```python
from build123d import *

# Parameters (mm, degrees)
F1_DEPTH = 152.4
F2_R     = 38.1
F3_DEPTH = 152.4
F5_DEPTH = 127
F7_DEPTH = 25.4


with BuildPart() as f1:
    # F0 (on Front) → F1 (new body)
    with BuildSketch(Plane.XZ):
        with BuildLine():
            Line((0, 50.8), (0, 0))
            Line((0, 0), (127, 0))
            Line((127, 0), (127, 154.6394254648))
            ThreePointArc((127, 154.6394254648), (84.2300226684, 178.0283138665), (80.8435975712, 226.6579672344))
            Line((80.8435975712, 226.6579672344), (0, 50.8))
        make_face()
        with BuildLine():
            Line((127, 154.6394254648), (127, 0))
            Line((127, 0), (254, 0))
            Line((254, 0), (254, 50.8))
            Line((254, 50.8), (173.1564024288, 226.6579672344))
            ThreePointArc((173.1564024288, 226.6579672344), (176.6255238934, 216.2997835762), (177.8, 205.4394254648))
            ThreePointArc((177.8, 205.4394254648), (162.9210244843, 169.5184009805), (127, 154.6394254648))
        make_face()
        with BuildLine():
            ThreePointArc((80.8435975712, 226.6579672344), (84.2300226684, 178.0283138665), (127, 154.6394254648))
            ThreePointArc((127, 154.6394254648), (162.9210244843, 169.5184009805), (177.8, 205.4394254648))
            ThreePointArc((177.8, 205.4394254648), (176.6255238934, 216.2997835762), (173.1564024288, 226.6579672344))
            ThreePointArc((173.1564024288, 226.6579672344), (127, 256.2394254648), (80.8435975712, 226.6579672344))
        make_face()
    extrude(amount=F1_DEPTH)

    # F2 (on face) → F3 (cut)
    with BuildSketch(Plane(origin=(0, 0, 0), x_dir=(-1, 0, 0), z_dir=(0, 1, 0))):
        with Locations((-127, 205.4394254648)):
            Circle(F2_R)
    extrude(amount=-F3_DEPTH, mode=Mode.SUBTRACT)

    # F4 (on face) → F5 (cut)
    with BuildSketch(Plane(origin=(0, 0, 0), x_dir=(-1, 0, 0), z_dir=(0, 1, 0))):
        with BuildLine():
            Line((-173.1564024288, 226.6579672344), (-254, 50.8))
            Line((-254, 50.8), (-139.7, 50.8))
            Line((-139.7, 50.8), (-139.7, 156.2525369679))
            ThreePointArc((-139.7, 156.2525369679), (-172.8830053448, 183.6359894848), (-173.1564024288, 226.6579672344))
        make_face()
        with BuildLine():
            Line((0, 50.8), (-80.8435975712, 226.6579672344))
            ThreePointArc((-80.8435975712, 226.6579672344), (-77.3744761066, 216.2997835762), (-76.2, 205.4394254648))
            ThreePointArc((-76.2, 205.4394254648), (-86.8390737159, 174.3309057314), (-114.3, 156.2525369679))
            Line((-114.3, 156.2525369679), (-114.3, 109.0697127324))
            Line((-114.3, 109.0697127324), (-114.3, 50.8))
            Line((-114.3, 50.8), (0, 50.8))
        make_face()
    extrude(amount=-F5_DEPTH, mode=Mode.SUBTRACT)

    # F6 (on face) → F7 (cut)
    with BuildSketch(Plane(origin=(0, 0, 0), x_dir=(-1, 0, 0), z_dir=(0, 1, 0))):
        with BuildLine():
            ThreePointArc((-114.3, 156.2525369679), (-127, 154.6394254648), (-139.7, 156.2525369679))
            Line((-139.7, 156.2525369679), (-139.7, 50.8))
            Line((-139.7, 50.8), (-114.3, 50.8))
            Line((-114.3, 50.8), (-114.3, 156.2525369679))
        make_face()
    extrude(amount=-F7_DEPTH, mode=Mode.SUBTRACT)


solid = f1.part
```
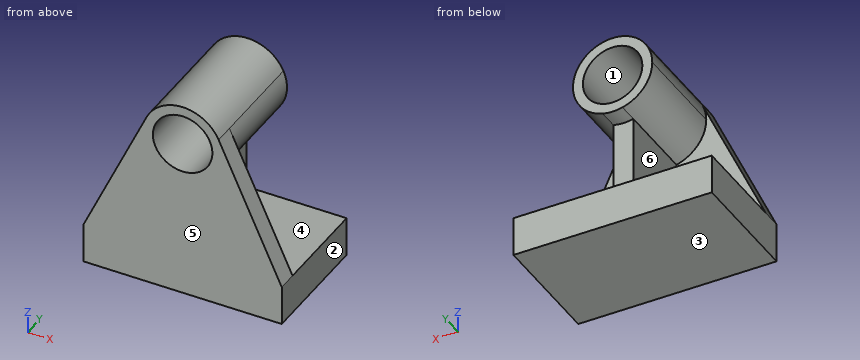
CAD build for the part. Positions are in the model's coordinates, mm. Face numbers are marked on the shaded views. A direction names the side the tool comes from. Coordinates: 2 decimals unless noted, no trailing zeros. Order: outer loops, then holes, each group sorted by start corner. A loop starts at its lowest first (then second) coordinate and runs counter-clockwise, first axis right, second up. Notation, with made-up numbers: (14.25, 16.25) -> (60.25, 16.25) arc R22 ccw to (60.25, 41.25) -> close; hole circle Ø2 at (41.25, 56.25). An arc over 180 degrees is marked (long way). Use one line per item in the form item = value. Start each with the question number.
1) Band-saw the part on A-A on x = 127. Give the cut face in (y, z), then the cut area to 3 significant figures.
2) Pull direction Z, two halves, no side cores. Call the marked faces 1, 2 and 3: +Z half, -Z half, draft (parallel to the pull), parting line (faces both ways), or undercut.
3) Band-saw the part on C-C on z = 197.5. Give the cut face in (x, y), then the cut area to 3 significant figures.
4) Band-saw the part on B-B on y = -136. Give the cut face in (x, z), then the cut area to 3 significant figures.
5) Drop flat-ended pins along their axis: pin 1 (3 mm diameter, centred on y = -73, z = 196, fed in from +X); pin 2 (4 mm diameter, centred on x = 132.5, z = 88, fed in from +Y); pin 3 (4 mm diameter, centred on x = 184, y = -60.5, fed in from +Z). Give the stop position or say it passes through.
6) Band-saw the part on D-D on y = -79. Give the cut face in (x, z), then the cut area to 3 significant figures.
7) Tool access for the marked faces 4, 5 and 6: list every direction of +Z, -Z, +X, -X, +Y, -Y with a clear straight run to the whole face (end or side of a thin tool).
8) Drill centre lines: L1, parallel to Z at x = 127, y = -45; L2, parallel to Z at x = 100.5, y = -103.5; L3, parallel to Z at x = 109.5, y = -124.5. Where is each one in solid material? Low to high. Write a range as [from, to].
Entries:
q1.outline = (-152.4, 0) -> (0, 0) -> (0, 50.8) -> (-25.4, 50.8) -> (-25.4, 154.64) -> (0, 154.64) -> (0, 167.34) -> (-152.4, 167.34) -> close; (-152.4, 243.54) -> (0, 243.54) -> (0, 256.24) -> (-152.4, 256.24) -> close
q1.area = 24,800 mm2
q2.face_1 = undercut
q2.face_2 = draft
q2.face_3 = -Z half
q3.outline = (67.44, -152.4) -> (89.74, -152.4) -> (89.74, 0) -> (76.82, 0) -> (76.82, -127) -> (67.44, -127) -> close; (164.26, -152.4) -> (186.56, -152.4) -> (186.56, -127) -> (177.18, -127) -> (177.18, 0) -> (164.26, 0) -> close
q3.area = 4,410 mm2
q4.outline = (0, 0) -> (254, 0) -> (254, 50.8) -> (173.16, 226.66) arc R50.8 ccw to (80.84, 226.66) -> (0, 50.8) -> close; hole circle Ø76.2 at (127, 205.44)
q4.area = 40,800 mm2
q5.pin_1 = 177.18
q5.pin_2 = -25.4
q5.pin_3 = 50.8
q6.outline = (0, 0) -> (254, 0) -> (254, 50.8) -> (139.7, 50.8) -> (139.7, 156.25) arc R50.8 ccw (long way) to (114.3, 156.25) -> (114.3, 50.8) -> (0, 50.8) -> close; hole circle Ø76.2 at (127, 205.44)
q6.area = 19,100 mm2
q7.face_4 = +Y
q7.face_5 = +Z, -Z, +X, -X, -Y
q7.face_6 = -X, +Y
q8.L1 = [0, 167.34], [243.54, 256.24]
q8.L2 = [0, 50.8], [162.1, 178.06], [232.81, 248.78]
q8.L3 = [0, 50.8], [157.75, 171.6], [239.28, 253.13]
